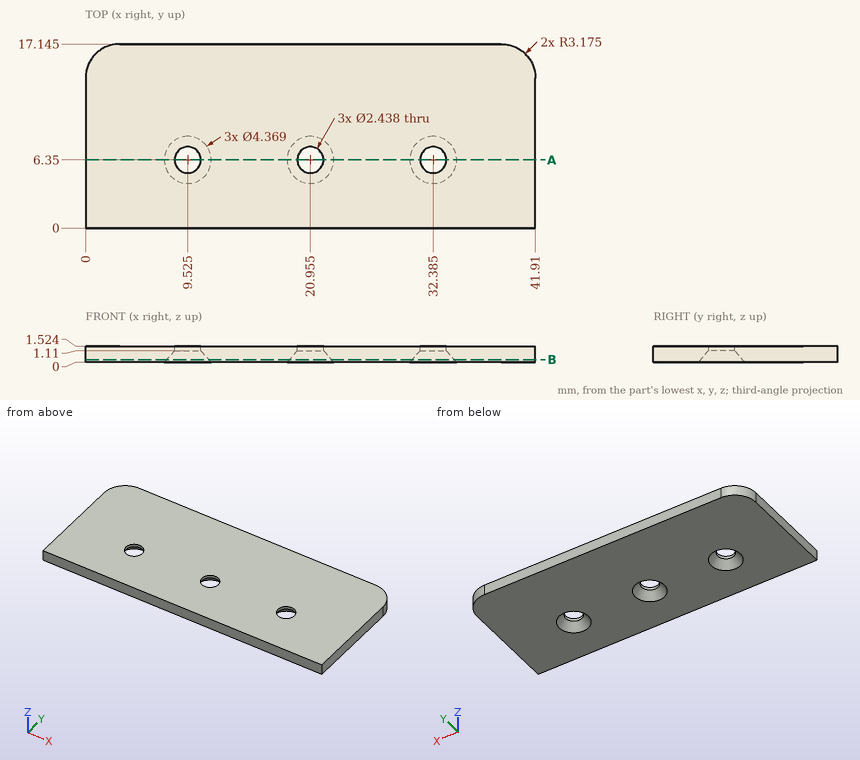
Can you work these out from the drawing? Everything is in mm from the part's minimum corner. Give positions to 0.01 mm unless a question says otherwise; leave off trailing zeros. Order: outer loops, then holes, each group sorted by start corner. A loop starts at its lowest first (then second) coordinate and runs counter-clockwise, first axis right, second up. Notation, with made-up numbers: M 29,79.5 L 60,79.5 A4 ccw 60,84.5 Z; hole C 56,-0.5 d1. An arc over 180 degrees is marked long. One line per question, with ' | ' between items.
1. If I drill on line 1 (X direction, y = 6.35, z = 1.35) (1 decimal); line 2 (Y direction, x = 9.5, z = 0.8) (1 decimal); line 3 (Y direction, x = 31.5, z = 1.2) (1 decimal), over which ranges is the centre line in solid material (lowest first)?
Results:
line 1: 0 to 8.3, 10.7 to 19.7, 22.2 to 31.2, 33.6 to 41.9 | line 2: 0 to 4.9, 7.8 to 17.1 | line 3: 0 to 5.5, 7.2 to 17.1
2. I want a section at A-A (y = 6.35). List the corners of the cut face in (x, z) for me (1 decimal).
Results:
outline: M 0,0 L 7.3,0 L 8.3,1.1 L 8.3,1.5 L 0,1.5 Z; M 10.7,1.1 L 11.7,0 L 18.8,0 L 19.7,1.1 L 19.7,1.5 L 10.7,1.5 Z; M 22.2,1.1 L 23.1,0 L 30.2,0 L 31.2,1.1 L 31.2,1.5 L 22.2,1.5 Z; M 33.6,1.1 L 34.6,0 L 41.9,0 L 41.9,1.5 L 33.6,1.5 Z
3. I want a section at B-B (z = 0.25). Give the number of separate pieces and of enclosed holes in the cut face, and give its area (3 significant figures).
Results:
separate pieces: 1 | enclosed holes: 3 | area: 678 mm²
4. I'm going to push a flat-ended pin straight in: pin 1 (3 mm diameter, centred on x = 9.525, y = 6.35, fed in from -Z). Where does the tip first touch, or does it pass through?
Results:
pin 1: z = 0.79
